Geometry: final body of the model. Coordinates: model frame, mm. Face numbers are marked on the shaded views. A direction names the side the tool comes from. Give positions to 0.01 mm unless a question says otherwise; leave off trailing zeros. Loops run counter-clockwise (first coordinate to the right, second up) from the corner with the lowest first, then second, coordinate; pieces in that order, holes last.
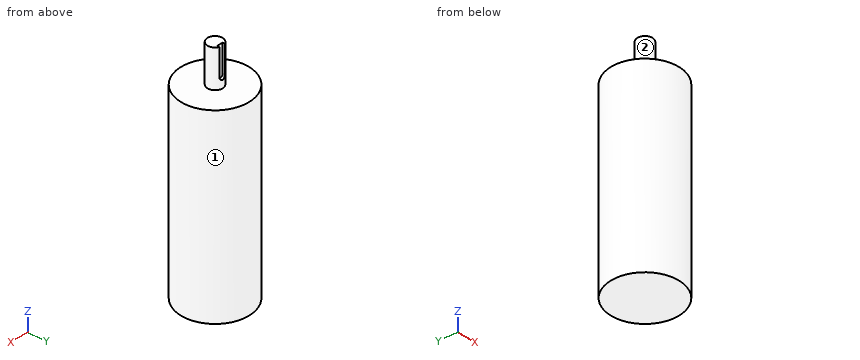
from build123d import *

# Parameters (mm, degrees)
SKETCH1_R           = 22.5
BOSS_EXTRUDE1_DEPTH = 125
SKETCH3_R           = 5
BOSS_EXTRUDE2_DEPTH = 25
CUT_EXTRUDE1_START  = -20
CUT_EXTRUDE1_DEPTH  = 20
FILLET1_R           = 2


with BuildPart() as part:
    # Sketch1 → Boss-Extrude1 (new body)
    with BuildSketch(Plane.XY):
        Circle(SKETCH1_R)
    extrude(amount=BOSS_EXTRUDE1_DEPTH)

    # Sketch3 → Boss-Extrude2 (add)
    with BuildSketch(Plane.XY.offset(125)):
        Circle(SKETCH3_R)
    extrude(amount=BOSS_EXTRUDE2_DEPTH)

    # Sketch4 → Cut-Extrude1 (cut)
    with BuildSketch(Plane.XY.offset(150).offset(CUT_EXTRUDE1_START)):
        with BuildLine():
            Line((-2, 3.184954178), (2, 3.184954178))
            Line((2, 3.184954178), (2, 4.582575695))
            ThreePointArc((2, 4.582575695), (0, 5), (-2, 4.582575695))
            Line((-2, 4.582575695), (-2, 3.184954178))
        make_face()
    extrude(amount=CUT_EXTRUDE1_DEPTH, mode=Mode.SUBTRACT)

    # Fillet1
    fillet1_edges = [part.edges().sort_by_distance(p)[0] for p in [
        (-2, 3.883764937, 130),
        (2, 3.883764937, 130),
    ]]
    fillet(fillet1_edges, radius=FILLET1_R - 0.0001)  # a hair under: the kernel refuses the full size


solid = part.part
Item 1: Section query D-D on y = -15. Return loops of the section in (x, z), plus the area to 3 significant figures.
Values follow:
outline: (-16.77, 0) - (16.77, 0) - (16.77, 125) - (-16.77, 125) - close
area: 4,190 mm2
Item 2: Set-up query: the marked faces 1 and 2. Return all of +Z, -Z, +X, -X, +Y, -Y with unobstructed straight access to the full face (end or side cutting, diameter ignored); none if empty.
Values follow:
face 1: +Z, -Z
face 2: +Z
Item 3: Pin query (flat end, axial travel): pin 1 (6 mm diameter, centred on y = 16.5, z = 95, fed in from -X); pin 2 (6 mm diameter, centred on y = 12, z = 101, fed in from +X); pin 3 (3 mm diameter, centred on y = 7.5, z = 78.5, fed in from +X). Return the tip coordinate at first contact, or that it passes through.
Values follow:
pin 1: stops at x = -18
pin 2: stops at x = 20.62
pin 3: stops at x = 21.69
Item 4: Ray query, probe 1 along Z at (x, y) = (7.5, 9); probe 2 along Y at (x, z) = (12, 32.5); probe 3 along Y at (x, z) = (-20.5, 17). Return the intervals inside material, ascending.
Values follow:
probe 1: z = 0 to 125
probe 2: y = -19.03 to 19.03
probe 3: y = -9.27 to 9.27
Item 5: Section query A-A on y = 0. Return loops of the section in (x, z), plus the area to 4 significant figures.
Values follow:
outline: (-22.5, 0) - (22.5, 0) - (22.5, 125) - (5, 125) - (5, 150) - (-5, 150) - (-5, 125) - (-22.5, 125) - close
area: 5,875 mm2
Item 6: Section query C-C on x = -7.5. Return loops of the section in (y, z).
Values follow:
outline: (-21.21, 0) - (21.21, 0) - (21.21, 125) - (-21.21, 125) - close
Item 7: Section query B-B on z = 121. Return loops of the section in (x, y).
Values follow:
outline: circle Ø45 at (0, 0)
